```python
from build123d import *

# Parameters (mm, degrees)
SKETCH1_R           = 60.957989534
BOSS_EXTRUDE1_DEPTH = 5
SKETCH1_4_R         = 60.957989534
SKETCH1_4_R_2       = 46.132101341
BOSS_EXTRUDE2_DEPTH = 30
FILLET2_R           = 10
FILLET3_R           = 10
FILLET5_R           = 3


with BuildPart() as part:
    # Sketch1 → Boss-Extrude1 (new body)
    with BuildSketch(Plane(origin=(0, 0, 0), x_dir=(1, 0, 0), z_dir=(0, 1, 0))):
        with Locations((-18.5585839, 19.037515097)):
            Circle(SKETCH1_R)
    extrude(amount=BOSS_EXTRUDE1_DEPTH)

    # Sketch1<4> → Boss-Extrude2 (add)
    with BuildSketch(Plane(origin=(0, 0, 0), x_dir=(1, 0, 0), z_dir=(0, 1, 0))):
        with Locations((-18.5585839, 19.037515097)):
            Circle(SKETCH1_4_R)
        with Locations((-18.5585839, 19.037515097)):
            Circle(SKETCH1_4_R_2, mode=Mode.SUBTRACT)
    extrude(amount=BOSS_EXTRUDE2_DEPTH)

    # Fillet2
    fillet2_edges = [part.edges().sort_by_distance(p)[0] for p in [
        (-64.69068524, 5, -19.037515097),
    ]]
    fillet(fillet2_edges, radius=FILLET2_R)

    # Fillet3
    fillet3_edges = [part.edges().sort_by_distance(p)[0] for p in [
        (-64.69068524, 30, -19.037515097),
    ]]
    fillet(fillet3_edges, radius=FILLET3_R)

    # Fillet5
    fillet5_edges = [part.edges().sort_by_distance(p)[0] for p in [
        (-79.516573434, 30, -19.037515097),
    ]]
    fillet(fillet5_edges, radius=FILLET5_R)


solid = part.part
```
Geometry check sheet. Reference: the model listing, model coordinates, mm. Round coordinates to 2 decimals unless told otherwise and drop trailing zeros. Loops run counter-clockwise (first coordinate to the right, second up) from the corner with the lowest first, then second, coordinate; pieces in that order, holes last. Notation, with made-up numbers: (70, -17) - (76, -17) arc R9 cw to (76, -1) - close; hole circle Ø1 at (-3.75, 65). An arc over 180 degrees is marked (long way). Write each question's results on one line, items separated by ' | '. Start each with the question number.
Q1. Cross-section at B-B on y = 2. Enter the section's corners in (x, z), and give its area (3 significant figures).
Q2. Thickness scan on line 1 (Y direction, x = -47, z = -36.5); line 2 (Z direction, x = -32.5, y = 22.5); line 3 (X direction, y = 20.75, z = -35). Record the ranges inside material, lowest first. Write a range as [from, to].
Q3. Release check for a two-part mould opening along Z. For faces 1 (the flat face through (-19, 0, -20)), 2 (the flat face through (-19, 5, -20)), 3 (the cylindrical face through (-31.77, 13.31, 40.47)), 4 (the cylindrical face through (25.443, 17.465, -32.894)) record: +Z half, -Z half, draft (parallel to the pull), parting line (faces both ways), or undercut.
Q4. Cross-section at C-C on y = 24.75. Enter the section's corners in (x, z).
Q5. Cross-section at A-A on y = 12.5. Enter the section's corners in (x, z), and give its area (3 significant figures).
Q6. Gauge pin test, flat ends, axial feed: P1, Ø10, axis at y = 23, z = 6, coming from the -X side; P2, Ø1.5, axis at x = 17.5, y = 9.5, coming from the -Z side; P3, Ø12, axis at y = 21.5, z = -6.5, coming from the -X side (3 decimals); P4, Ø8, axis at x = -12, z = -34.5, coming from the -Y side. Record the tip position at first contact, or that the pin passes through.
Answers below:
1) outline: circle Ø121.92 at (-18.56, -19.04) | area: 11,700 mm²
2) line 1: y = [0, 5] | line 2: z = [-78.38, -63.35], [25.27, 40.3] | line 3: x = [-77.39, -61.87], [24.75, 40.27]
3) face 1: draft | face 2: undercut | face 3: parting line | face 4: undercut
4) outline: circle Ø121.92 at (-18.56, -19.04); hole circle Ø94.66 at (-18.56, -19.04)
5) outline: circle Ø121.92 at (-18.56, -19.04); hole circle Ø91.63 at (-18.56, -19.04) | area: 5,080 mm²
6) P1: stops at x = -76.13 | P2: stops at z = -68.73 | P3: stops at x = -79.165 | P4: stops at y = 0
